Geometry: see drawing. Coordinates: mm, zero at the bounding-box minimum. A direction names the side the tool comes from. Give positions to 0.01 mm unless a question says otherwise; leave off trailing zeros. Loops run counter-clockwise (first coordinate to the right, second up) from the corner with the lowest first, then second, coordinate; pieces in that order, holes last. Notation, with made-up numbers: M -10,-28.75 L 15,-28.75 A19 ccw 15,-9.75 Z; hole C 21,-19 d4. An arc over 180 degrees is marked long. Return JSON: item names as keys, results as strings. Group by question number.
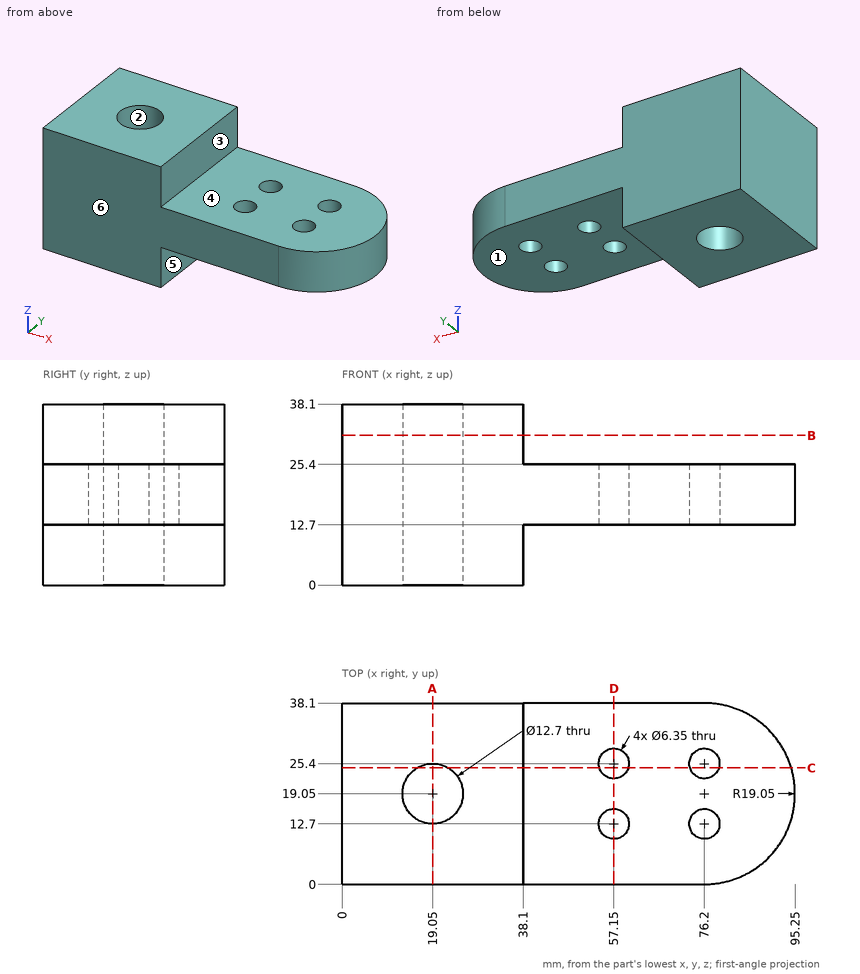
Item 1: Section A-A, the plane x = 19.05. Return loops of the section in (y, z).
Item 2: First-contact query: pin 1 Ø10 at (y, z) = (14.5, 33.5) entering from +X; pin 2 Ø3 at (y, z) = (6.5, 12.5) entering from +X; pin 3 Ø19 at (x, y) = (74, 23) entering from +Z. Flat tips, straight axial feed; report the tip coordinate or a pass-through.
Item 3: Section C-C, the plane y = 24.5. Return loops of the section in (x, z), then the cut area to 3 significant figures.
Item 4: Pull-direction query (X, two-part tool) for the marked faces 1, 2 and 3; classes: pulls with the +X half, pulls with the -X half, needs draft (parallel to the pull), parting line crosses it, or undercut.
Item 5: Material intervals for line 1 (Y direction, x = 76, z = 20); line 2 (Y direction, x = 19, z = 22), sorted ascending. Write a range as from..to.
Item 6: Section D-D, the plane x = 57.15. Return loops of the section in (y, z) (3 decimals), then the cut area to 3 significant figures.
Item 7: Reachability of the marked faces 4, 5 and 6 from +Z, -Z, +X, -X, +Y, -Y: full face, straight path, thin tool, end or side. Return the list, or none.
Item 8: Section B-B, the plane z = 31.5. Return loops of the section in (x, y), then the cut area to 3 significant figures.
Answer below:
{
 "1": {"outline": "M 0,0 L 12.7,0 L 12.7,38.1 L 0,38.1 Z; M 25.4,0 L 38.1,0 L 38.1,38.1 L 25.4,38.1 Z"},
 "2": {"pin 1": "x = 38.1", "pin 2": "x = 91.71", "pin 3": "z = 25.4"},
 "3": {"outline": "M 0,0 L 15.79,0 L 15.79,38.1 L 0,38.1 Z; M 22.31,0 L 38.1,0 L 38.1,12.7 L 54.11,12.7 L 54.11,25.4 L 38.1,25.4 L 38.1,38.1 L 22.31,38.1 Z; M 60.19,12.7 L 73.16,12.7 L 73.16,25.4 L 60.19,25.4 Z; M 79.24,12.7 L 94.45,12.7 L 94.45,25.4 L 79.24,25.4 Z", "area": "1,760 mm^2"},
 "4": {"face 1": "needs draft", "face 2": "undercut", "face 3": "pulls with the +X half"},
 "5": {"line 1": "0..9.53, 15.87..22.23, 28.57..38.1", "line 2": "0..12.7, 25.4..38.1"},
 "6": {"outline": "M 0,12.7 L 9.525,12.7 L 9.525,25.4 L 0,25.4 Z; M 15.875,12.7 L 22.225,12.7 L 22.225,25.4 L 15.875,25.4 Z; M 28.575,12.7 L 38.1,12.7 L 38.1,25.4 L 28.575,25.4 Z", "area": "323 mm^2"},
 "7": {"face 4": "+Z, +X, +Y, -Y", "face 5": "-Z, +X, +Y, -Y", "face 6": "+Z, -Z, +X, -X, -Y"},
 "8": {"outline": "M 0,0 L 38.1,0 L 38.1,38.1 L 0,38.1 Z; hole C 19.05,19.05 d12.7", "area": "1,320 mm^2"}
}
